Job drawing, mm, ordinate dimensions from the low corner. One solid piece. A direction names the side the tool comes from. Round coordinates to 2 decimals unless told otherwise and drop trailing zeros. Write each loop counter-clockwise with the first axis right and the second up, starting at its lowest first coordinate (ties: lowest second). Pieces come first, ordered by that corner, then holes. Notation, with made-up numbers: (-17, 69.25) -> (22, 69.25) arc R26 ccw to (22, 100.25) -> close; hole circle Ø4 at (49, 23.25). An arc over 180 degrees is marked (long way). Use CSV: the item, a comma, the result in double quotes. Start each with the question number.
(1) Two-plate mould, pull along Y, no slides. Class the marked faces 3, 4, 5 and 6: released by +Y, released by -Y, zero draft, split by the parting line, or undercut.
(2) Saw through at C-C (x = 69.75). Give the cut face in (y, z).
(3) Saw through at A-A (y = 15.5). Give the cut face in (x, z) (3 decimals).
(4) Which spindle directions (+Z, -Z, +X, -X, +Y, -Y) get a long thin tool onto all of the face, cutting with end or side? Do the marked faces 1 and 2. Say none if no direction does.
(5) Drop flat-ended pins along their axis: pin 1 (6 mm diameter, centred on x = 64.5, y = 25.5, fed in from +Z); pin 2 (2.5 mm diameter, centred on x = 59.425, y = 15.5, fed in from -Z); pin 3 (4 mm diameter, centred on x = 65, y = 25, fed in from +Z). Give the stop position or say it passes through.
(6) Probe line 1 (X direction, y = 15.5, z = 2.65) (3 decimals); line 2 (Y direction, x = 34.5, z = 22.25); line 3 (Z direction, x = 67, y = 25.5). List the from-to ranges inside material, lowest first. Write a range as [from, to].
(7) Saw through at D-D (x = 12). Give the cut face in (y, z).
(8) Saw through at B-B (z = 21.5). Give the cut face in (x, y).
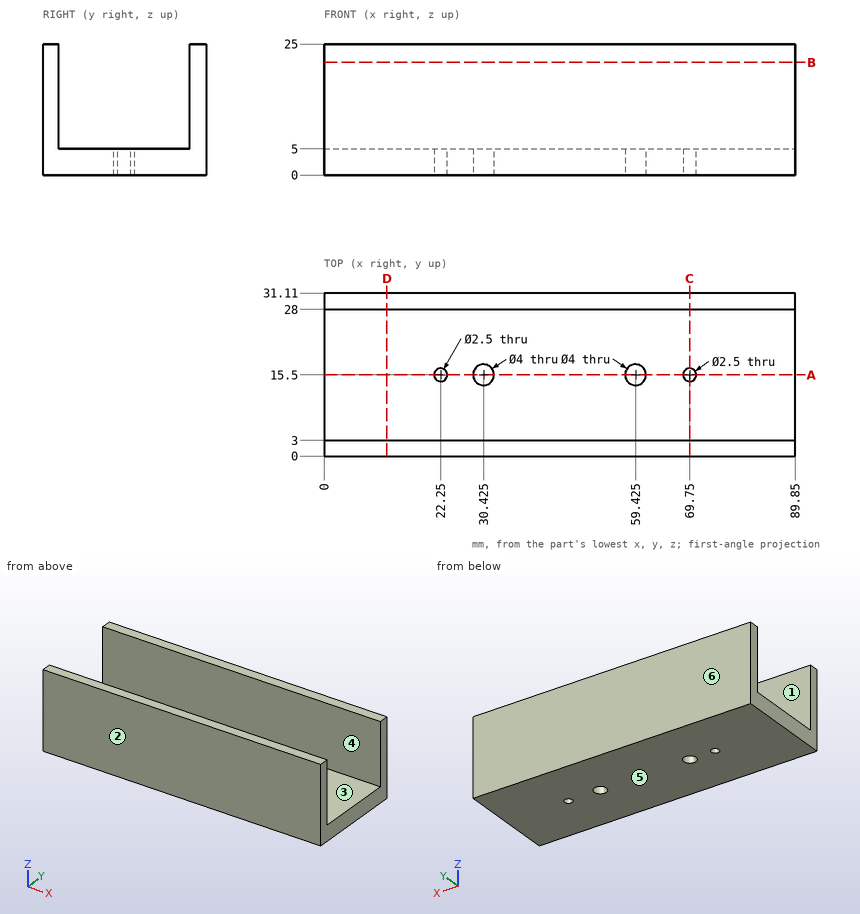
Answers:
1,face 3,"undercut"
1,face 4,"undercut"
1,face 5,"zero draft"
1,face 6,"released by +Y"
2,outline,"(0, 0) -> (14.25, 0) -> (14.25, 5) -> (3, 5) -> (3, 25) -> (0, 25) -> close; (16.75, 0) -> (31.11, 0) -> (31.11, 25) -> (28, 25) -> (28, 5) -> (16.75, 5) -> close"
3,outline,"(0, 0) -> (21, 0) -> (21, 5) -> (0, 5) -> close; (23.5, 0) -> (28.425, 0) -> (28.425, 5) -> (23.5, 5) -> close; (32.425, 0) -> (57.425, 0) -> (57.425, 5) -> (32.425, 5) -> close; (61.425, 0) -> (68.5, 0) -> (68.5, 5) -> (61.425, 5) -> close; (71, 0) -> (89.85, 0) -> (89.85, 5) -> (71, 5) -> close"
4,face 1,"+Z, +X, -X"
4,face 2,"+Z, -Z, +X, -X, -Y"
5,pin 1,"stops at z = 25"
5,pin 2,"passes through"
5,pin 3,"stops at z = 5"
6,line 1,"x = [0, 21], [23.5, 28.425], [32.425, 57.425], [61.425, 68.5], [71, 89.85]"
6,line 2,"y = [0, 3], [28, 31.11]"
6,line 3,"z = [0, 5]"
7,outline,"(0, 0) -> (31.11, 0) -> (31.11, 25) -> (28, 25) -> (28, 5) -> (3, 5) -> (3, 25) -> (0, 25) -> close"
8,outline,"(0, 0) -> (89.85, 0) -> (89.85, 3) -> (0, 3) -> close; (0, 28) -> (89.85, 28) -> (89.85, 31.11) -> (0, 31.11) -> close"
